from build123d import *

# Parameters (mm, degrees)
F0_W     = 400
F0_H     = 400
F1_DEPTH = 38.1
F2_SIZE  = 38.1
F3_W     = 203.2
F3_H     = 203.2
F4_DEPTH = 510


with BuildPart() as f1:
    # F0 (on Top) → F1 (new body)
    with BuildSketch(Plane.XY):
        Rectangle(F0_W, F0_H)
    extrude(amount=F1_DEPTH)

    # F2
    f2_edges = [f1.edges().sort_by_distance(p)[0] for p in [
        (-200, 200, 19.05),
        (-200, -200, 19.05),
        (200, -200, 19.05),
        (200, 200, 19.05),
    ]]
    chamfer(f2_edges, length=F2_SIZE)

    # F3 (on face) → F4 (join)
    with BuildSketch(Plane.XY.offset(38.1)):
        Rectangle(F3_W, F3_H)
    extrude(amount=F4_DEPTH)


solid = f1.part
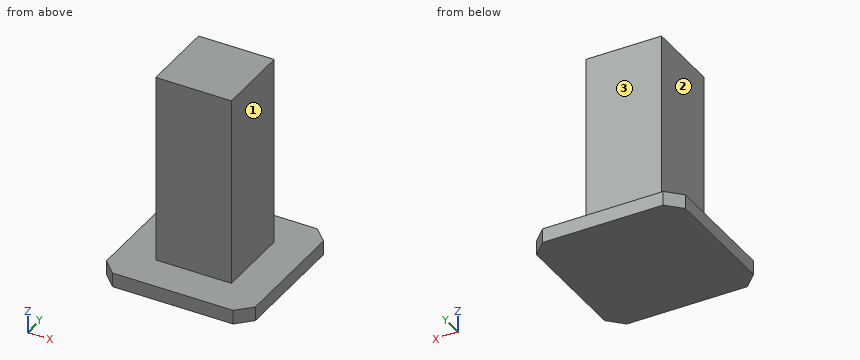
The model under review builds one solid part; all positions refer to its coordinate system, in mm. Face numbers are marked on the shaded views. A direction names the side the tool comes from. Coordinates: 2 decimals unless noted, no trailing zeros. Loops run counter-clockwise (first coordinate to the right, second up) from the corner with the lowest first, then second, coordinate; pieces in that order, holes last. Notation, with made-up numbers: (-5, -14.5) -> (39, -14.5) arc R19 ccw to (39, -0.5) -> close; hole circle Ø11 at (-15.5, 51). An arc over 180 degrees is marked (long way). Use a Markdown table: item, result. Add a question column.
1. Add section C-C on z = 47. Write out the cut boundary in (x, y), plus the area to 3 significant figures.
2. Add section D-D on y = -134.5. Write out the cut boundary in (x, z).
3. Machinability: for the marked faces 1, 2 and 3, which of the approach directions +Z, -Z, +X, -X, +Y, -Y give a long, thin tool a straight path to every point of the face, cutting with its end or side? Answer none if there is none.
4. Clearance check with flat-ended pins moving along their axes: pin 1 Ø3 at (x, z) = (93.5, 176.5) entering from +Y; pin 2 Ø4 at (y, z) = (-70, 181.5) entering from +X; pin 3 Ø10 at (x, y) = (154.5, 117) entering from +Z. State where each tip first meets the part, or that it passes through.
5. Add section A-A on y = 60. Write out the cut boundary in (x, z), plus the area to 3 significant figures.
6. To check wall thickness, follow line 1 (Y direction, x = -87, z = 449); line 2 (Z direction, x = -134.5, y = 60.5). State the ranges of each line that lie inside material, in increasing order.
Returned:
| question | item | result |
|---|---|---|
| 1 | outline | (-101.6, -101.6) -> (101.6, -101.6) -> (101.6, 101.6) -> (-101.6, 101.6) -> close |
| 1 | area | 41,300 mm² |
| 2 | outline | (-200, 0) -> (200, 0) -> (200, 38.1) -> (-200, 38.1) -> close |
| 3 | face 1 | +Z, +X, +Y, -Y |
| 3 | face 2 | +Z, -X, +Y, -Y |
| 3 | face 3 | +Z, +X, -X, +Y |
| 4 | pin 1 | stops at y = 101.6 |
| 4 | pin 2 | stops at x = 101.6 |
| 4 | pin 3 | stops at z = 38.1 |
| 5 | outline | (-200, 0) -> (200, 0) -> (200, 38.1) -> (101.6, 38.1) -> (101.6, 548.1) -> (-101.6, 548.1) -> (-101.6, 38.1) -> (-200, 38.1) -> close |
| 5 | area | 119,000 mm² |
| 6 | line 1 | y = -101.6 to 101.6 |
| 6 | line 2 | z = 0 to 38.1 |
